Verification items for the finished model (mm, model axes). A direction names the side the tool comes from. Round coordinates to 2 decimals unless told otherwise and drop trailing zeros. Write each loop counter-clockwise with the first axis right and the second up, starting at its lowest first coordinate (ties: lowest second). Pieces come first, ordered by that corner, then holes. Notation, with made-up numbers: (63.5, 71) - (70.5, 71) arc R23 cw to (70.5, 103) - close; hole circle Ø11 at (18.25, -33.5). An arc over 180 degrees is marked (long way). Write each question's results on one line, items separated by ' | '.
```python
from build123d import *

# Parameters (mm, degrees)
SKETCH1_W           = 60
SKETCH1_H           = 14
BOSS_EXTRUDE1_DEPTH = 30
SKETCH2_W           = 3
SKETCH2_H           = 20
CUT_EXTRUDE1_DEPTH  = 45.676615807
CUT_EXTRUDE2_DEPTH  = 68.446274916


with BuildPart() as part:
    # Sketch1 → Boss-Extrude1 (new body)
    with BuildSketch(Plane(origin=(0, 0, 0), x_dir=(1, 0, 0), z_dir=(0, 1, 0))):
        Rectangle(SKETCH1_W, SKETCH1_H)
    extrude(amount=BOSS_EXTRUDE1_DEPTH)

    # Sketch2 → Cut-Extrude1 (cut, through all)
    with BuildSketch(Plane.XY.offset(7)):
        with Locations((-22.5, 10)):
            Rectangle(SKETCH2_W, SKETCH2_H)
        with Locations((22.5, 10)):
            Rectangle(SKETCH2_W, SKETCH2_H)
    extrude(amount=-CUT_EXTRUDE1_DEPTH, mode=Mode.SUBTRACT)

    # Sketch3 → Cut-Extrude2 (cut, through all)
    with BuildSketch(Plane.ZY.offset(30)):
        Polygon((-7, 30), (-5, 0), (-7, 0), align=None)
        Polygon((7, 30), (5, 0), (7, 0), align=None)
    extrude(amount=-CUT_EXTRUDE2_DEPTH, mode=Mode.SUBTRACT)


solid = part.part
```
(1) Mould release check, pull along X, two halves, no side actions. Record for faces 1 (the flat face through (24, 10, 0)), 2 (the flat face through (0, 30, 0)), 3 (the flat face through (30, 15, 0)): released by +X, released by -X, zero draft, split by the parting line, or undercut.
Answer:
face 1: undercut | face 2: zero draft | face 3: released by +X
(2) Go/stop test with flat-tipped pins: pin 1 Ø2 at (x, y) = (17.5, 15.5) entering from +Z; pin 2 Ø0.9 at (x, z) = (-22, -0.5) entering from -Y; pin 3 Ø3 at (x, y) = (-4, 6.5) entering from -Z. Record where each tip stops, or that it passes through.
Answer:
pin 1: z = 6.1 | pin 2: y = 20 | pin 3: z = -5.53
(3) Thickness scan on L1, parallel to X at y = 11.5, z = -4.5; L2, parallel to Y at x = -22.5, z = 1; L3, parallel to Z at x = 3.5, y = 18. Record the ranges inside material, lowest first.
Answer:
L1: -30 to -24, -21 to 21, 24 to 30 | L2: 20 to 30 | L3: -6.2 to 6.2
(4) Set-up check for faces 4 (the flat face through (-27, 0, 0)), 5 (the flat face through (-24, 10, 0)): record each of +Z, -Z, +X, -X, +Y, -Y from which the full face is reachable in a straight line by a thin tool's end or side.
Answer:
face 4: +Z, -Z, +X, -X, -Y | face 5: +Z, -Z, -Y
(5) Section check A-A (y = 15). Record the cut outline in (x, z).
Answer:
outline: (-30, -6) - (-24, -6) - (-24, 6) - (-30, 6) - close; (-21, -6) - (21, -6) - (21, 6) - (-21, 6) - close; (24, -6) - (30, -6) - (30, 6) - (24, 6) - close
(6) Section check B-B (z = -1.5). Record the cut outline in (x, y).
Answer:
outline: (-30, 0) - (-24, 0) - (-24, 20) - (-21, 20) - (-21, 0) - (21, 0) - (21, 20) - (24, 20) - (24, 0) - (30, 0) - (30, 30) - (-30, 30) - close
(7) Section check D-D (x = -16.5). Record the cut outline in (y, z).
Answer:
outline: (0, -5) - (30, -7) - (30, 7) - (0, 5) - close
(8) Section check C-C (y = 2). Record the cut outline in (x, z).
Answer:
outline: (-30, -5.13) - (-24, -5.13) - (-24, 5.13) - (-30, 5.13) - close; (-21, -5.13) - (21, -5.13) - (21, 5.13) - (-21, 5.13) - close; (24, -5.13) - (30, -5.13) - (30, 5.13) - (24, 5.13) - close
